```python
from build123d import *

# Parameters (mm, degrees)
F0_W           = 30
F0_H           = 24
F1_DEPTH       = 3
F2_D           = 3.3
F3_R           = 8
F4_DEPTH       = 16
F6_W           = 2.2
F6_H           = 5.6
F10_D          = 5.5
F11_R          = 5
F12_W          = 35.0341517478
F12_H          = 6.4177829772
F13_DEPTH      = 25
F13_DEPTH_BACK = 25


with BuildPart() as f1:
    # F0 (on Top) → F1 (new body)
    with BuildSketch(Plane.XY):
        Rectangle(F0_W, F0_H)
    extrude(amount=-F1_DEPTH)

    # F2 (through all)
    with Locations(Plane.XY):
        with Locations((-9, 6.7), (9, 6.7)):
            Hole(F2_D / 2)

    # F3 (on face) → F4 (join)
    with BuildSketch(Plane.XY):
        Circle(F3_R)
    extrude(amount=F4_DEPTH)

    # F6 (on Front) → F8 (revolve, cut)
    with BuildSketch(Plane.XZ):
        with Locations((-6.9275095962, 9.7)):
            Rectangle(F6_W, F6_H)
    revolve(axis=Axis((0, 0, 17.9499220103), (0, 0, 1)), mode=Mode.SUBTRACT)

    # F10 (through all)
    with Locations(Plane(origin=(0, 0, -3), x_dir=(1, 0, 0), z_dir=(0, 0, -1))):
        with Locations((0, 0)):
            Hole(F10_D / 2)

    # F11
    f11_edges = [f1.edges().sort_by_distance(p)[0] for p in [
        (15, -12, -1.5),
        (15, 12, -1.5),
        (-15, 12, -1.5),
        (-15, -12, -1.5),
    ]]
    fillet(f11_edges, radius=F11_R)

    # F12 (on Front) → F13 (cut, two sides)
    with BuildSketch(Plane.XZ) as f13_sk:
        with Locations((-0.1057451591, -3.2088914886)):
            Rectangle(F12_W, F12_H)
    extrude(amount=-F13_DEPTH, mode=Mode.SUBTRACT)
    extrude(f13_sk.sketch, amount=F13_DEPTH_BACK, mode=Mode.SUBTRACT)


solid = f1.part
```
CAD build for the part. Positions are in the model's coordinates, mm. A direction names the side the tool comes from. Coordinates: 2 decimals unless noted, no trailing zeros. Write each loop counter-clockwise with the first axis right and the second up, starting at its lowest first coordinate (ties: lowest second). Pieces come first, ordered by that corner, then holes.
(1) Cut at D-D, the plane x = -3.25. List the corners of the cut face in (y, z).
(2) Two-plate mould, pull along Z, no slides. Class faces 1 (the face through (0.596, 2.685, 8.112)), 2 (the face through (-1, 6, 12.5)), 3 (the face through (3, 0, 0)): +Z half, -Z half, draft (parallel to the pull), parting line (faces both ways), or undercut.
(3) Cut at C-C, the plane z = 15. List the corners of the cut face in (x, y).
(4) 3-axis set-ups, long thin cutter, end or side, ignore diameter. For faces 4 (the face through (-1, 6, 6.9)), 5 (the face through (3, 0, 16)): which of +Z, -Z, +X, -X, +Y, -Y reach the whole face in a straight line?
(5) Flat gauge pins, fed straight in: pin 1 (8 mm diameter, centred on x = -5, z = 7, fed in from +Y); pin 2 (9 mm diameter, centred on x = 0, y = 0, fed in from -Z); pin 3 (1 mm diameter, centred on x = 4.5, z = 7.5, fed in from -Y); pin 4 (1 mm diameter, centred on y = -3.5, z = 8.5, fed in from +X). Where does each tip first touch, or does it go through?
(6) Drill centre lines: probe 1 along Z at (x, y) = (-5.25, -3); probe 2 along Y at (x, z) = (0, 4.5); probe 3 along Y at (x, z) = (0, 10.75). Where is each one in solid material? Low to high.
(7) Cut at A-A, the plane y = 0. List the corners of the cut face in (x, z), and give its area (3 significant figures).
Geometry says:
1. outline: (-7.31, 0) - (7.31, 0) - (7.31, 6.9) - (4.84, 6.9) - (4.84, 12.5) - (7.31, 12.5) - (7.31, 16) - (-7.31, 16) - (-7.31, 12.5) - (-4.84, 12.5) - (-4.84, 6.9) - (-7.31, 6.9) - close
2. face 1: draft
2. face 2: undercut
2. face 3: -Z half
3. outline: circle Ø16 at (0, 0); hole circle Ø5.5 at (0, 0)
4. face 4: none
4. face 5: +Z, +X, -X, +Y, -Y
5. pin 1: stops at y = 7.94
5. pin 2: stops at z = 0
5. pin 3: stops at y = -4.24
5. pin 4: stops at x = 5
6. probe 1: z = 0 to 6.9, 12.5 to 16
6. probe 2: y = -8 to -2.75, 2.75 to 8
6. probe 3: y = -5.83 to -2.75, 2.75 to 5.83
7. outline: (-8, 0) - (-2.75, 0) - (-2.75, 16) - (-8, 16) - (-8, 12.5) - (-5.83, 12.5) - (-5.83, 6.9) - (-8, 6.9) - close; (2.75, 0) - (8, 0) - (8, 6.9) - (5.83, 6.9) - (5.83, 12.5) - (8, 12.5) - (8, 16) - (2.75, 16) - close
7. area: 144 mm2
